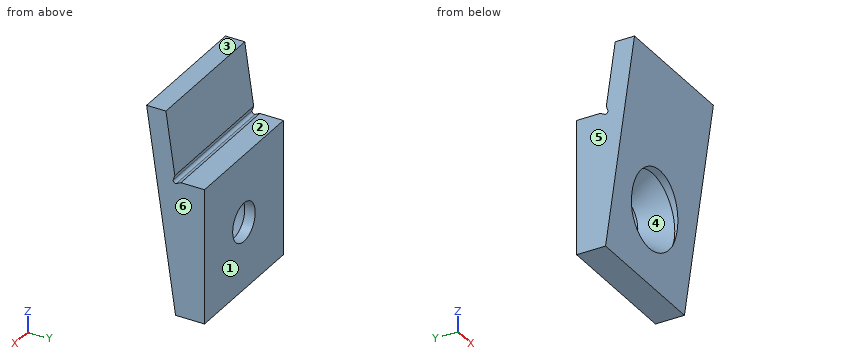
```python
from build123d import *

# Parameters (mm, degrees)
SKETCH003_R     = 1.75
SKETCH004_R     = 4
SKETCH005_R     = 4
PAD001_DEPTH    = 2
PAD_DEPTH       = 7
SKETCH001_R     = 0.25
POCKET_DEPTH    = 14.001
SKETCH002_R     = 2
POCKET001_DEPTH = 6.001
CHAMFER_SIZE    = 0.3


with BuildPart() as obj1:
    # Sketch003 → Loft section 0
    with BuildSketch(Plane.XZ.offset(-0.75)):
        Circle(SKETCH003_R)
    # Sketch004 → Loft section 1
    with BuildSketch(Plane.XZ.offset(2.25)):
        Circle(SKETCH004_R)
    loft()

    # Sketch005 → Pad001 (new body)
    with BuildSketch(Plane.XZ.offset(2.25)):
        Circle(SKETCH005_R)
    extrude(amount=PAD001_DEPTH)


with BuildPart() as halterung_unten:
    # Sketch → Pad (new body, symmetric)
    with BuildSketch(Plane.YZ):
        Polygon((-4.5, 14), (-2.5, 14), (-1.5, 7), (1.5, 7), (1.5, -7), (-1.5, -7), align=None)
    extrude(amount=PAD_DEPTH, both=True)

    # Sketch001 → Pocket (cut, through all)
    with BuildSketch(Plane.YZ.offset(7)):
        with Locations((-1.5, 7)):
            Circle(SKETCH001_R)
    extrude(amount=-POCKET_DEPTH, mode=Mode.SUBTRACT)

    # Sketch002 → Pocket001 (cut, through all)
    with BuildSketch(Plane.ZX.offset(1.5)):
        Circle(SKETCH002_R)
    extrude(amount=-POCKET001_DEPTH, mode=Mode.SUBTRACT)

    # Cut: cut obj1
    add(obj1.part, mode=Mode.SUBTRACT)

    # Chamfer
    chamfer_edges = [halterung_unten.edges().sort_by_distance(p)[0] for p in [
        (0, -1.535355, 7.247487),
        (0, -1.25, 7),
    ]]
    chamfer(chamfer_edges, length=CHAMFER_SIZE)


solid = halterung_unten.part
```
Here's how the part is built. I have some questions about the finished solid (model axes, mm). Face numbers are marked on the shaded views. A direction names the side the tool comes from. Give positions to 0.01 mm unless a question says otherwise; leave off trailing zeros. Order: outer loops, then holes, each group sorted by start corner. A loop starts at its lowest first (then second) coordinate and runs counter-clockwise, first axis right, second up. Notation, with made-up numbers: M 63,20.5 L 82,20.5 A7 ccw 82,28.5 Z; hole C -39,81 d1. An arc over 180 degrees is marked long. Use a Markdown table: item, result. Add a question column.
1. Suppose I cut it at B-B (x = 0). List the corners of the cut face in (y, z) for me.
2. For pin 1 Ø3 at (x, y) = (2, -2) entering from +Z; pin 2 Ø1.5 at (x, y) = (5, -0.5) entering from +Z; pin 3 Ø4 at (x, z) = (3, 8.5) entering from -Y; pin 4 Ø6.5 at (x, z) = (0, 0) entering from -Y, each with a flat end and sliding along its axis, tell me the tip position at first contact or that it passes through.
3. On a 3-axis mill with a long thin cutter (end or side, diameter ignored), from which of +Z, -Z, +X, -X, +Y, -Y can I reach the whole of each face in a straight line? I mean the marked faces 1 and 2. Say none if no direction works.
4. Suppose I cut it at C-C (y = -0.5). List the corners of the cut face in (x, z) for me (1 decimal).
5. Suppose I cut it at D-D (y = -4). List the corners of the cut face in (x, z) for me.
6. If we mould it in two halves opening along X, with no side actions, what happens to the marked faces 3, 4, 5 and 6? For each: +X half, -X half, draft (parallel to the pull), parting line (faces both ways), or undercut.
7. I need wall thicknesses on probe 1 along X at (y, z) = (0.95, 0); probe 2 along Z at (x, y) = (-2.75, 1). Which ranges of each line are inside material? Lowest first, please. Write a range as from..to.
8. Suppose I cut it at A-A (x = -5). List the corners of the cut face in (y, z) for me, and give its area (3 significant figures).
Results list:
| question | item | result |
|---|---|---|
| 1 | outline | M -4.5,14 L -3.07,4 L -2.25,4 L 0.42,2 L 1.5,2 L 1.5,7 L -0.95,7 L -1.43,6.76 A0.25 cw -1.75,7.04 L -1.58,7.54 L -2.5,14 Z; M -1.96,-3.78 L -1.5,-7 L 1.5,-7 L 1.5,-2 L 0.42,-2 Z |
| 2 | pin 1 | stops at z = 14 |
| 2 | pin 2 | stops at z = 7 |
| 2 | pin 3 | stops at y = -4 |
| 2 | pin 4 | stops at y = -1.25 |
| 3 | face 1 | +Z, -Z, +X, -X, +Y |
| 3 | face 2 | +Z, +X, -X, +Y |
| 4 | outline | M -7,-7 L 7,-7 L 7,7 L -7,7 Z; hole C 0,0 d5.4 |
| 5 | outline | M -7,10.5 L 7,10.5 L 7,14 L -7,14 Z |
| 6 | face 3 | draft |
| 6 | face 4 | undercut |
| 6 | face 5 | -X half |
| 6 | face 6 | +X half |
| 7 | probe 1 | x = -7..-2, 2..7 |
| 7 | probe 2 | z = -7..7 |
| 8 | outline | M -4.5,14 L -1.5,-7 L 1.5,-7 L 1.5,7 L -0.95,7 L -1.43,6.76 A0.25 cw -1.75,7.04 L -1.58,7.54 L -2.5,14 Z |
| 8 | area | 69.8 mm² |
